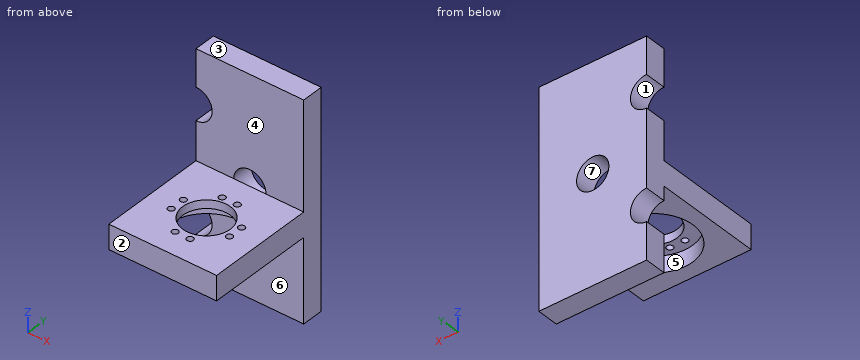
from build123d import *

# Parameters (mm, degrees)
F0_W      = 10
F0_H      = 20
F1_DEPTH  = 2
F2_R      = 1.5
F3_DEPTH  = 25.4
F4_W      = 10
F4_H      = 2.271716
F5_DEPTH  = 10
F6_R      = 1.5
F7_DEPTH  = 2
F8_R      = 3.65
F9_DEPTH  = 1.5
F10_R     = 2.211105
F11_DEPTH = 1
F12_R     = 0.3
F13_DEPTH = 1


with BuildPart() as f1:
    # F0 (on Front) → F1 (new body)
    with BuildSketch(Plane.XZ):
        Rectangle(F0_W, F0_H)
    extrude(amount=F1_DEPTH)

    # F2 (on face) → F3 (cut)
    with BuildSketch(Plane.XZ.offset(2)):
        with Locations((-5, 5.06894)):
            Circle(F2_R)
        with Locations((-5, -5.06894)):
            Circle(F2_R)
    extrude(amount=-F3_DEPTH, mode=Mode.SUBTRACT)

    # F4 (on face) → F5 (join)
    with BuildSketch(Plane.XZ.offset(2)):
        with Locations((0, -1.135858)):
            Rectangle(F4_W, F4_H)
    extrude(amount=F5_DEPTH)

    # F6 (on face) → F7 (cut)
    with BuildSketch(Plane(origin=(0, 0, 0), x_dir=(-1, 0, 0), z_dir=(0, 1, 0))):
        Circle(F6_R)
    extrude(amount=-F7_DEPTH, mode=Mode.SUBTRACT)

    # F8 (on face) → F9 (cut)
    with BuildSketch(Plane(origin=(0, 0, -2.271716), x_dir=(1, 0, 0), z_dir=(0, 0, -1))):
        with Locations((0, 6.969983)):
            Circle(F8_R)
    extrude(amount=-F9_DEPTH, mode=Mode.SUBTRACT)

    # F10 (on face) → F11 (cut)
    with BuildSketch(Plane(origin=(0, 0, -0.771716), x_dir=(1, 0, 0), z_dir=(0, 0, -1))):
        with Locations((0, 6.969983)):
            Circle(F10_R)
    extrude(amount=-F11_DEPTH, mode=Mode.SUBTRACT)

    # F12 (on face) → F13 (cut)
    with BuildSketch(Plane(origin=(0, 0, -0.771716), x_dir=(1, 0, 0), z_dir=(0, 0, -1))):
        with Locations((0.7, 4.309839)):
            Circle(F12_R)
        with Locations((-0.7, 4.309839)):
            Circle(F12_R)
        with Locations((0.7, 9.71972)):
            Circle(F12_R)
        with Locations((-0.7, 9.71972)):
            Circle(F12_R)
        with Locations((-2.693097, 6.302936)):
            Circle(F12_R)
        with Locations((-2.693097, 7.702936)):
            Circle(F12_R)
        with Locations((2.716784, 6.302936)):
            Circle(F12_R)
        with Locations((2.716784, 7.702936)):
            Circle(F12_R)
    extrude(amount=-F13_DEPTH, mode=Mode.SUBTRACT)


solid = f1.part
The listing builds one solid part. Answer for the finished solid, in the listing's coordinates (mm). Face numbers are marked on the shaded views. A direction names the side the tool comes from. Coordinates: 2 decimals unless noted, no trailing zeros. Order: outer loops, then holes, each group sorted by start corner. A loop starts at its lowest first (then second) coordinate and runs counter-clockwise, first axis right, second up.
Q1. Given P1, Ø2, axis at x = -2.5, z = 4.5, coming from the -Y side; P2, Ø3, axis at x = 2.5, y = -7.5, coming from the -Z side; P3, Ø1, axis at x = 2, y = -6, coming from the -Z side, each flat-ended and moving along its own axis, determine where each tip first touches the part or whether it passes through.
Q2. A cutting plane is placed at C-C, the plane y = -5. Write down the section's boundary in (x, z), and give its area (3 significant figures).
Q3. Which of the six approach directions +Z, -Z, +X, -X, +Y, -Y give full straight-line access (tool end or side, diameter ignored) to the marked faces 4, 5, 6 and 7?
Q4. For a pull along Z with two mould halves and no side action, classify the marked faces 1, 2 and 3 as pulls with the +Z half, pulls with the -Z half, needs draft (parallel to the pull), parting line crosses it, or undercut.
Q5. Consider line 1 (Y direction, x = 0, z = -1.8); line 2 (Y direction, x = 0, z = -1.35); line 3 (Y direction, x = -0.7, z = -0.35). Determine where each line is inside the solid, lowest interval first.
Q6. A cutting plane is placed at D-D, the plane z = -3. Write down the section's boundary in (x, y).
Q7. A cutting plane is placed at A-A, the plane x = 0. Write down the section's boundary in (y, z).
Q8. A cutting plane is placed at B-B, the plane y = -1. Write down the section's boundary in (x, z).
Answers follow:
1. P1: stops at y = -2
1. P2: stops at z = -2.27
1. P3: stops at z = -0.77
2. outline: (-5, -2.27) - (-3.07, -2.27) - (-3.07, -0.77) - (-1, -0.77) - (-1, 0) - (-5, 0) - close; (1, -0.77) - (3.07, -0.77) - (3.07, -2.27) - (5, -2.27) - (5, 0) - (1, 0) - close
2. area: 11.9 mm2
3. face 4: +Z, +X, -X, -Y
3. face 5: -Z
3. face 6: -Z, +X, -X, -Y
3. face 7: +Y
4. face 1: undercut
4. face 2: needs draft
4. face 3: pulls with the +Z half
5. line 1: y = -12 to -10.62, -3.32 to 0
5. line 2: y = -12 to -10.62, -3.32 to -2
5. line 3: y = -12 to -10.02, -9.42 to -9.07, -4.87 to -4.61, -4.01 to -2
6. outline: (-5, -2) - (5, -2) - (5, 0) - (-5, 0) - close
7. outline: (-12, -2.27) - (-10.62, -2.27) - (-10.62, -0.77) - (-9.18, -0.77) - (-9.18, 0) - (-12, 0) - close; (-4.76, -0.77) - (-3.32, -0.77) - (-3.32, -2.27) - (-2, -2.27) - (-2, -10) - (0, -10) - (0, -1.5) - (-2, -1.5) - (-2, 0) - (-4.76, 0) - close; (-2, 1.5) - (0, 1.5) - (0, 10) - (-2, 10) - close
8. outline: (-5, -10) - (5, -10) - (5, 10) - (-5, 10) - (-5, 6.57) arc R1.5 cw to (-5, 3.57) - (-5, -3.57) arc R1.5 cw to (-5, -6.57) - close; hole circle Ø3 at (0, 0)
